Could you check a few things on this model? Use its own coordinates, in mm. A direction names the side the tool comes from. Give positions to 0.01 mm unless a question says otherwise; leave off trailing zeros. Order: outer loops, then holes, each group sorted by start corner. A loop starts at its lowest first (then second) coordinate and runs counter-clockwise, first axis right, second up. Notation, with made-up numbers: (16, -21.5) -> (43, -21.5) arc R14 ccw to (43, -3.5) -> close; hole circle Ø10 at (32, -20). An arc over 180 degrees is marked (long way). One line per item, written item: value.
```python
from build123d import *

# Parameters (mm, degrees)
SKETCH1_R           = 14
BOSS_EXTRUDE1_DEPTH = 1.7
CIRPATTERN1_COUNT   = 6
FILLET1_R           = 0.25


with BuildPart() as part:
    # Sketch1 → Boss-Extrude1 (new body)
    with BuildSketch(Plane(origin=(0, 0, 0), x_dir=(1, 0, 0), z_dir=(0, 1, 0))):
        with Locations(Location((0, 0, 0), (0, 0, 270))):
            Circle(SKETCH1_R)
    extrude(amount=BOSS_EXTRUDE1_DEPTH)

    # Sketch14 → CBORE for M5 Hex Head Bolt1 (revolve, cut)
    with BuildSketch(Plane(origin=(-11, 1.7, 0), x_dir=(0, 0, 1), z_dir=(1, 0, 0))):
        Polygon((0, 0), (0, 5.660946681), (1.1, 5), (1.1, 1.3), (2.6, 1.3), (2.6, 0), align=None)
    cbore_for_m5_hex_head_bolt1 = revolve(axis=Axis((-11, 8.05, 0), (0, -1, 0)), mode=Mode.SUBTRACT)

    # CirPattern1: CBORE for M5 Hex Head Bolt1 ×6 about axis
    cirpattern1_axis = Axis((0, 0, 0), (0, 1, 0))
    for i in range(1, CIRPATTERN1_COUNT):
        add(cbore_for_m5_hex_head_bolt1.rotate(cirpattern1_axis, i * 360 / CIRPATTERN1_COUNT), mode=Mode.SUBTRACT)

    # Fillet1
    fillet1_edges = [part.edges().sort_by_distance(p)[0] for p in [
        (-3.24833395, 0.4, -10.826279442),
        (7.75166605, 0.4, -8.226279442),
        (-11, 0.4, -2.6),
    ]]
    fillet(fillet1_edges, radius=FILLET1_R)


solid = part.part
```
1) Suppose I cut it at B-B, the plane x = 11. Write out the boundary of the cut face in (y, z), then the cut area to 3 significant figures.
Answer below:
outline: (0, -8.66) -> (1.7, -8.66) -> (1.7, -2.6) -> (0.4, -2.6) -> (0.4, -1.1) -> (0, -1.1) -> close; (0, 1.1) -> (0.4, 1.1) -> (0.4, 2.6) -> (1.7, 2.6) -> (1.7, 8.66) -> (0, 8.66) -> close
area: 21.8 mm2
2) Suppose I cut it at C-C, the plane x = -5.5. Write out the boundary of the cut face in (y, z), then the cut area to 3 significant figures.
Answer below:
outline: (0, -12.87) -> (1.7, -12.87) -> (1.7, -12.13) -> (0.65, -12.13) arc R0.25 cw to (0.4, -11.88) -> (0.4, -10.63) -> (0, -10.63) -> close; (0, -8.43) -> (0.4, -8.43) -> (0.4, -7.18) arc R0.25 cw to (0.65, -6.93) -> (1.7, -6.93) -> (1.7, 6.93) -> (0.4, 6.93) -> (0.4, 8.43) -> (0, 8.43) -> close; (0, 10.63) -> (0.4, 10.63) -> (0.4, 12.13) -> (1.7, 12.13) -> (1.7, 12.87) -> (0, 12.87) -> close
area: 28.5 mm2
3) Suppose I cut it at D-D, the plane y = 1.25. Write out the boundary of the cut face in (x, z), then the cut area to 3 significant figures.
Answer below:
outline: circle Ø28 at (0, 0); hole circle Ø5.2 at (-11, 0); hole circle Ø5.2 at (-5.5, -9.53); hole circle Ø5.2 at (-5.5, 9.53); hole circle Ø5.2 at (5.5, -9.53); hole circle Ø5.2 at (5.5, 9.53); hole circle Ø5.2 at (11, 0)
area: 488 mm2
4) We'd pull the mould along X, two halves only. Please class faces 1 (the cylindrical face through (5.39, 1.06, 6.93)), 2 (the flat face through (0, 0, 0)): +X half, -X half, draft (parallel to the pull), parting line (faces both ways), or undercut.
Answer below:
face 1: undercut
face 2: draft
5) For P1, Ø4.5, axis at x = -5.5, z = 9.53, coming from the +Y side, with a flat end and sliding along its axis, tell me the tip position at first contact or that it passes through.
Answer below:
P1: stops at y = 0.4
6) Suppose I cut it at A-A, the plane z = 0. Write out the boundary of the cut face in (x, y).
Answer below:
outline: (-14, 0) -> (-12.1, 0) -> (-12.1, 0.4) -> (-13.35, 0.4) arc R0.25 cw to (-13.6, 0.65) -> (-13.6, 1.7) -> (-14, 1.7) -> close; (-9.9, 0) -> (9.9, 0) -> (9.9, 0.4) -> (8.4, 0.4) -> (8.4, 1.7) -> (-8.4, 1.7) -> (-8.4, 0.65) arc R0.25 cw to (-8.65, 0.4) -> (-9.9, 0.4) -> close; (12.1, 0) -> (14, 0) -> (14, 1.7) -> (13.6, 1.7) -> (13.6, 0.4) -> (12.1, 0.4) -> close
7) For faces 3 (the flat face through (-4, 0.4, -10)), 4 (the cylindrical face through (-5.921, 0.203, -10.542)), which set-ups out of +Z, -Z, +X, -X, +Y, -Y let a thin tool reach every point of the face, with its end or its side?
Answer below:
face 3: +Y
face 4: +Y, -Y
8) If I drill on line 1 along X through (y, z) = (1.55, 0); line 2 along X through (y, z) = (0.3, 0); line 3 along Z through (x, y) = (7.5, 1.3), over which ranges is the centre line in solid material (lowest first)?
Answer below:
line 1: x = -14 to -13.6, -8.4 to 8.4, 13.6 to 14
line 2: x = -14 to -12.1, -9.9 to 9.9, 12.1 to 14
line 3: z = -11.82 to -11.19, -7.86 to 7.86, 11.19 to 11.82
